from build123d import *

# Parameters (mm, degrees)
SZKIC1_R                    = 11
SZKIC1_R_2                  = 2.5
DODANIE_WYCI_GNI_CIE1_DEPTH = 2
SZKIC2_R                    = 1.5
WYTNIJ_WYCI_GNI_CIE2_DEPTH  = 3
SZKIC3_OUTSIDE_W            = 88.13
SZKIC3_OUTSIDE_H            = 58.13
WYTNIJ_WYCI_GNI_CIE3_DEPTH  = 3


with BuildPart() as part:
    # Szkic1 → Dodanie-wyciągnięcie1 (new body)
    with BuildSketch(Plane.XY):
        with BuildLine():
            Line((-32, -20), (32, -20))
            ThreePointArc((32, -20), (34.121320344, -19.121320344), (35, -17))
            Line((35, -17), (35, 17))
            ThreePointArc((35, 17), (34.121320344, 19.121320344), (32, 20))
            Line((32, 20), (-32, 20))
            ThreePointArc((-32, 20), (-34.121320344, 19.121320344), (-35, 17))
            Line((-35, 17), (-35, -17))
            ThreePointArc((-35, -17), (-34.121320344, -19.121320344), (-32, -20))
        make_face()
        Circle(SZKIC1_R, mode=Mode.SUBTRACT)
        with Locations((-27, 14.666666667)):
            Circle(SZKIC1_R_2, mode=Mode.SUBTRACT)
        with BuildLine():
            ThreePointArc((27.662313373, -8.536108756), (29.93756488, -2.199008421), (31.480810618, 4.354921901))
            ThreePointArc((31.480810618, 4.354921901), (29.452911679, 7.251061728), (26.556771853, 5.223162789))
            ThreePointArc((26.556771853, 5.223162789), (25.143466206, -0.778931698), (23.059789106, -6.582453114))
            ThreePointArc((23.059789106, -6.582453114), (24.384223418, -9.860543068), (27.662313373, -8.536108756))
        make_face(mode=Mode.SUBTRACT)
        with BuildLine():
            ThreePointArc((-28.085714286, -16.981382282), (-24.496074307, -16.900850402), (-20.93862552, -16.414477411))
            ThreePointArc((-20.93862552, -16.414477411), (-18.963380552, -13.482173315), (-21.895684648, -11.506928346))
            ThreePointArc((-21.895684648, -11.506928346), (-24.891430995, -11.916505602), (-27.914285714, -11.984321922))
            ThreePointArc((-27.914285714, -11.984321922), (-30.49853018, -14.397137816), (-28.085714286, -16.981382282))
        make_face(mode=Mode.SUBTRACT)
    extrude(amount=DODANIE_WYCI_GNI_CIE1_DEPTH)

    # Szkic2 → Wytnij-wyciągnięcie2 (cut, through all)
    with BuildSketch(Plane.XY):
        with Locations((-10.606601718, 10.606601718)):
            Circle(SZKIC2_R)
        with Locations((10.606601718, 10.606601718)):
            Circle(SZKIC2_R)
        with Locations((10.606601718, -10.606601718)):
            Circle(SZKIC2_R)
        with Locations((-10.606601718, -10.606601718)):
            Circle(SZKIC2_R)
    extrude(amount=WYTNIJ_WYCI_GNI_CIE2_DEPTH, mode=Mode.SUBTRACT)

    # Szkic3 outside → Wytnij-wyciągnięcie3 (cut, through all)
    with BuildSketch(Plane.XY):
        Rectangle(SZKIC3_OUTSIDE_W, SZKIC3_OUTSIDE_H)
        with BuildLine():
            Line((32.464358731, -11.108986267), (34.865595884, 9.966401743))
            ThreePointArc((34.865595884, 9.966401743), (34.232704788, 12.173555294), (32.224489958, 13.286726951))
            Line((32.224489958, 13.286726951), (-26.396249527, 19.965716564))
            ThreePointArc((-26.396249527, 19.965716564), (-27, 20), (-27.603750473, 19.965716564))
            Line((-27.603750473, 19.965716564), (-32.571609752, 19.399700495))
            ThreePointArc((-32.571609752, 19.399700495), (-33.247974324, 19.241713465), (-33.869879413, 18.932419111))
            ThreePointArc((-33.869879413, 18.932419111), (-34.450895793, 18.337181113), (-34.723108417, 17.551185823))
            Line((-34.723108417, 17.551185823), (-34.948574845, 15.572292377))
            ThreePointArc((-34.948574845, 15.572292377), (-35, 14.666666667), (-34.948574845, 13.761040957))
            Line((-34.948574845, 13.761040957), (-31.363806409, -17.702067807))
            ThreePointArc((-31.363806409, -17.702067807), (-31.101077058, -18.632320729), (-30.556161181, -19.430734091))
            ThreePointArc((-30.556161181, -19.430734091), (-30.098141008, -19.761880936), (-29.551624806, -19.905966855))
            ThreePointArc((-29.551624806, -19.905966855), (-26.310608357, -19.993144599), (-23.075621923, -19.777157663))
            Line((-23.075621923, -19.777157663), (29.823252805, -13.750092193))
            ThreePointArc((29.823252805, -13.750092193), (31.604963507, -12.890696969), (32.464358731, -11.108986267))
        make_face(mode=Mode.SUBTRACT)
    extrude(amount=WYTNIJ_WYCI_GNI_CIE3_DEPTH, mode=Mode.SUBTRACT)


solid = part.part
Model file for the job. Use its own axes, mm. A direction names the side the tool comes from. Give positions to 0.01 mm unless a question says otherwise; leave off trailing zeros. Loops run counter-clockwise (first coordinate to the right, second up) from the corner with the lowest first, then second, coordinate; pieces in that order, holes last.
Item 1: Slice it at A-A (y = 0). Write the cut outline in (x, z), plus the area to 3 significant figures.
Check values:
outline: (-33.38, 0) - (-11, 0) - (-11, 2) - (-33.38, 2) - close; (11, 0) - (25.37, 0) - (25.37, 2) - (11, 2) - close; (30.54, 0) - (33.73, 0) - (33.73, 2) - (30.54, 2) - close
area: 79.9 mm2
Item 2: Drill centre lines: line 1 along Y through (x, z) = (-27, 0.75); line 2 along X through (y, z) = (-1, 0.85); line 3 along X through (y, z) = (-2.5, 0.9). Where is each one in solid material? Low to high.
Check values:
line 1: y = -20 to -17, -12 to 12.17, 17.17 to 20
line 2: x = -33.27 to -10.95, 10.95 to 25.08, 30.28 to 33.62
line 3: x = -33.1 to -10.71, 10.71 to 24.6, 29.85 to 33.45
Item 3: Which spindle directions (+Z, -Z, +X, -X, +Y, -Y) get a long thin tool onto all of the face, cutting with end or side? Do faces 1 (the face through (-34.445, 18.347, 0.986)), 2 (the face through (25.168, -0.696, 0.986)). Say none if no direction does.
Check values:
face 1: +Z, -Z, -X, +Y
face 2: +Z, -Z
Item 4: Slice it at C-C (x = 0). Write the cut outline in (y, z), plus the area to 3 significant figures.
Check values:
outline: (-17.15, 0) - (-11, 0) - (-11, 2) - (-17.15, 2) - close; (11, 0) - (16.96, 0) - (16.96, 2) - (11, 2) - close
area: 24.2 mm2
Item 5: Slice it at B-B (z = 1.65). Give the number of separate pieces and of enclosed holes in the cut face, plus the area to 3 significant figures.
Check values:
separate pieces: 1
enclosed holes: 8
area: 1,700 mm2
Item 6: Slice it at D-D (y = -5.5). Write the cut outline in (x, z), plus the area to 3 significant figures.
Check values:
outline: (-32.75, 0) - (-9.53, 0) - (-9.53, 2) - (-32.75, 2) - close; (9.53, 0) - (23.51, 0) - (23.51, 2) - (9.53, 2) - close; (28.85, 0) - (33.1, 0) - (33.1, 2) - (28.85, 2) - close
area: 82.9 mm2
Item 7: Drop a flat-ended pin along its axis: P1, Ø1, axis at y = 0, z = 1, coming from the -X side. Give the stop position or say it passes through.
Check values:
P1: stops at x = -33.44
Item 8: Mould opens along Y. For faces 3 (the face through (-9.8, 11.87, 0.99)), 4 (the face through (29.91, -2.29, 0.99)), 5 (the face through (-34.834, 16.576, 0.986)), 6 (the face through (3.004, -16.806, 0.986)) say: +Y half, -Y half, draft (parallel to the pull), parting line (faces both ways), or undercut.
Check values:
face 3: undercut
face 4: undercut
face 5: +Y half
face 6: -Y half
